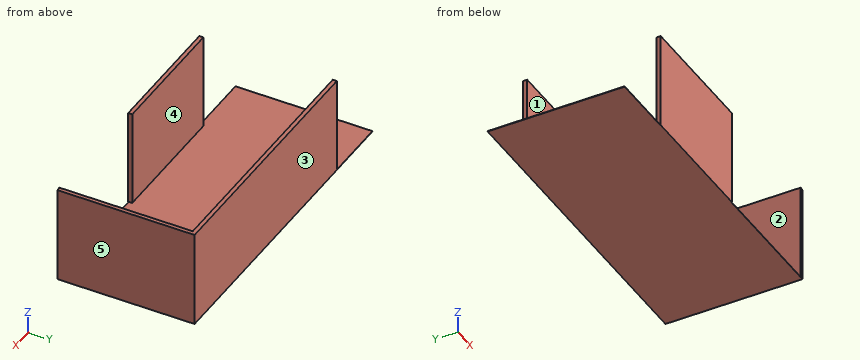
```python
from build123d import *

# Parameters (mm, degrees)
BOSS_EXTRUDE1_DEPTH   = 152.4
SKETCH1_W             = 203.2
SKETCH1_H             = 6.35
BOSS_EXTRUDE1_2_DEPTH = 152.4
SKETCH3_W             = 508
SKETCH3_H             = 215.132857965
BOSS_EXTRUDE2_DEPTH   = 0.635


with BuildPart() as part:
    # Sketch1 → Boss-Extrude1 (new body)
    with BuildSketch(Plane.XY):
        Polygon((400.096509451, -209.55), (406.4, -208.782857965), (406.4, 6.35), (0, 6.35), (0, 0), (400.096509451, 0), align=None)
    extrude(amount=BOSS_EXTRUDE1_DEPTH)



with BuildPart() as body_2:
    # Sketch1 → Boss-Extrude1 2 (new body)
    with BuildSketch(Plane.XY):
        with Locations((101.6, -206.375)):
            Rectangle(SKETCH1_W, SKETCH1_H)
    extrude(amount=BOSS_EXTRUDE1_2_DEPTH)


with BuildPart() as part_1:
    add(part.part)

    add(body_2.part)  # Boss-Extrude2 merges body 2
    # Sketch3 → Boss-Extrude2 (add)
    with BuildSketch(Plane(origin=(0, 0, 0), x_dir=(-1, 0, 0), z_dir=(0, 0, -1))):
        with Locations((-152.4, -101.216428983)):
            Rectangle(SKETCH3_W, SKETCH3_H)
    extrude(amount=-BOSS_EXTRUDE2_DEPTH)


solid = part_1.part
```
Here's how the part is built. I have some questions about the finished solid (model axes, mm). Face numbers are marked on the shaded views. A direction names the side the tool comes from. Coordinates: 2 decimals unless noted, no trailing zeros. Loops run counter-clockwise (first coordinate to the right, second up) from the corner with the lowest first, then second, coordinate; pieces in that order, holes last. Notation, with made-up numbers: (37, 79) - (56, 79) arc R11 ccw to (56, 98) - close; hole circle Ø7 at (-20.75, -20). An arc over 180 degrees is marked (long way). Return JSON: item names as keys, results as strings. Group by question number.
Item 1: If we section it at A-A on z = 24: Write out the boundary of the cut face in (x, y).
Item 2: We'd pull the mould along Y, two halves only. Please class the marked faces 1, 2 and 3: +Y half, -Y half, draft (parallel to the pull), parting line (faces both ways), or undercut.
Item 3: On a 3-axis mill with a long thin cutter (end or side, diameter ignored), from which of +Z, -Z, +X, -X, +Y, -Y can I reach the whole of each face in a straight line? I mean the marked faces 4 and 5. Say none if no direction works.
Item 4: If we section it at B-B on x = 30: Write out the boundary of the cut face in (y, z) (3 decimals), and give its area (3 significant figures).
Item 5: Will these pins go through, and if not, where does the flat tip stop? P1, Ø12, axis at x = 316, y = -26, coming from the -Z side; P2, Ø5, axis at y = -205, z = 109, coming from the -X side; P3, Ø5, axis at x = 340.5, z = 59.5, coming from the -Y side; P4, Ø2, axis at y = -159, z = 116, coming from the -X side.
Item 6: If we section it at D-D on x = 251: Write out the boundary of the cut face in (y, z) (3 decimals), and give its area (3 significant figures).
Item 7: If we section it at C-C on y = -27: Write out the boundary of the cut face in (x, z) (1 decimal), and give its area (3 significant figures).
Item 8: I need wall thicknesses on line 1 (Y direction, x = 186.5, z = 92); line 2 (Z direction, x = -53.5, y = -111) (3 decimals); line 3 (Y direction, x = 317.5, z = 77). Which ranges of each line are inside material? Lowest first, please. Write a range as from..to.
Calculated:
{
 "1": {"outline": "(0, -209.55) - (203.2, -209.55) - (203.2, -203.2) - (0, -203.2) - close; (0, 0) - (400.1, 0) - (400.1, -209.55) - (406.4, -208.78) - (406.4, 6.35) - (0, 6.35) - close"},
 "2": {"face 1": "undercut", "face 2": "draft", "face 3": "+Y half"},
 "3": {"face 4": "+Z, -X", "face 5": "+Z, -Z, +X, +Y, -Y"},
 "4": {"outline": "(-209.55, 0) - (6.35, 0) - (6.35, 152.4) - (0, 152.4) - (0, 0.635) - (-203.2, 0.635) - (-203.2, 152.4) - (-209.55, 152.4) - close", "area": "2,060 mm^2"},
 "5": {"P1": "stops at z = 0", "P2": "stops at x = 0", "P3": "stops at y = 0", "P4": "stops at x = 400.1"},
 "6": {"outline": "(-208.783, 0) - (6.35, 0) - (6.35, 152.4) - (0, 152.4) - (0, 0.635) - (-208.783, 0.635) - close", "area": "1,100 mm^2"},
 "7": {"outline": "(-101.6, 0) - (406.4, 0) - (406.4, 152.4) - (400.1, 152.4) - (400.1, 0.6) - (-101.6, 0.6) - close", "area": "1,280 mm^2"},
 "8": {"line 1": "y = -209.55..-203.2, 0..6.35", "line 2": "z = 0..0.635", "line 3": "y = 0..6.35"}
}
